Can you work these out from the model? Positions are in its coordinate system, mm. A direction names the side the tool comes from. Give positions to 0.01 mm unless a question says otherwise; leave off trailing zeros. Order: outer loops, then holes, each group sorted by start corner. A loop starts at its lowest first (then second) coordinate and runs counter-clockwise, first axis right, second up.
Item 1: Which directions (+Z, -Z, +X, -X, +Y, -Y) give clear straight access to the entire face, cutting with the end or side of a thin tool? Please do faces 4 (the cylindrical face through (7, -6, 0)), 5 (the flat face through (14.16, 0, -3)), 6 (the flat face through (8.16, -1, -1)).
Item 2: If I drill on line 1 along Z through (x, y) = (6.5, 0); line 2 along X through (y, z) = (-4, -4.75); line 3 along Z through (x, y) = (2.5, 0), over which ranges is the centre line in solid material (lowest first)?
Item 3: I'm going to push flat-ended pins straight in: pin 1 Ø8 at (x, z) = (2, -3.5) entering from +Y; pin 2 Ø6 at (x, y) = (4, 5.5) entering from -Z. Where does each tip first touch, or does it pass through?
Item 4: I want a section at D-D, the plane x = 8.5. Write out the boundary of the cut face in (y, z), then the cut area to 3 significant figures.
Item 5: If we mould it in two halves opening along Y, with no side actions, what happens to faces 1 (the cylindrical face through (11.38, 7.573, 2.385)), 2 (the cylindrical face through (11.2, -0.54, -2.44)), 3 (the flat face through (9.4, 5, -4))? For each: +Y half, -Y half, draft (parallel to the pull), parting line (faces both ways), or undercut.
Item 6: I want a section at C-C, the plane x = 5.5. Write out the boundary of the cut face in (y, z), then the cut area to 3 significant figures.
```python
from build123d import *

# Parameters (mm, degrees)
F2_SIZE = 1


# Not quite as in the source:
# - a fillet or chamfer that OpenCascade refuses, or shapes differently, is made with other operations: its cross-section is extruded or revolved along the edge and cut away or added


with BuildPart() as f1:
    # F0 (on Top) → F1 (revolve)
    with BuildSketch(Plane.XY):
        Polygon((0, 7.94), (0, 1), (8.16, 1), (8.16, 2.5), (14.16, 2.5), (14.16, 7.94), (9.4, 7.94), (9.4, 6), (4.76, 6), (4.76, 7.94), align=None)
    revolve(axis=Axis((7.08, 0, 0), (1, 0, 0)))

    # F2
    f2_edges = [f1.edges().sort_by_distance(p)[0] for p in [
        (0, -7.94, 0),
        (14.16, -7.94, 0),
        (0, -1, 0),
    ]]
    chamfer(f2_edges, length=F2_SIZE)

    # F3: chamfer of 0.25 on 3 edges, made by hand

    # F3_s1 → F3_t2 (revolve, cut)
    with BuildSketch(Plane.XY):
        Polygon((4.51, 7.94), (4.76, 7.69), (4.76, 7.94), align=None)
    revolve(axis=Axis((4.76, 0, 0), (1, 0, 0)), mode=Mode.SUBTRACT)

    # F3_s3 → F3_t4 (revolve, cut)
    with BuildSketch(Plane.XY):
        Polygon((9.4, 7.69), (9.65, 7.94), (9.4, 7.94), align=None)
    revolve(axis=Axis((9.4, 0, 0), (1, 0, 0)), mode=Mode.SUBTRACT)

    # F3_s5 → F3_t6 (revolve, cut)
    with BuildSketch(Plane.XY):
        Polygon((0, 2.1035533906), (0.0732233047, 1.9267766953), (0, 2), align=None)
    revolve(axis=Axis((0, 0, 0), (1, 0, 0)), mode=Mode.SUBTRACT)


solid = f1.part
```
Results list:
1. face 4: none
1. face 5: +Z, -Z, +X, +Y, -Y
1. face 6: +X
2. line 1: z = -6 to -1, 1 to 6
2. line 2: x = 0 to 4.76, 9.4 to 14.16
2. line 3: z = -7.94 to -1, 1 to 7.94
3. pin 1: stops at y = 7.94
3. pin 2: stops at z = -7.54
4. outline: circle Ø12 at (0, 0); hole circle Ø5 at (0, 0)
4. area: 93.5 mm2
5. face 1: parting line
5. face 2: undercut
5. face 3: draft
6. outline: circle Ø12 at (0, 0); hole circle Ø2 at (0, 0)
6. area: 110 mm2
